from build123d import *

# Parameters (mm, degrees)
F3_DEPTH  = 5
F5_DEPTH  = 15
F6_W      = 2
F6_H      = 3
F7_DEPTH  = 20.5
F8_W      = 3
F8_H      = 1
F9_DEPTH  = 17.5068136575
F10_R     = 0.3
F11_R     = 0.1
F12_R     = 0.1
F13_W     = 100
F13_H     = 100
F14_DEPTH = 46.1004730675


with BuildPart() as f2:
    # F1 (on Front) → F2 (revolve)
    with BuildSketch(Plane.XZ):
        with BuildLine():
            Line((-2, 62), (-10, 62))
            add(Edge.make_bspline(
                [(-10, 62), (-11.8174263966, 57.1809415466), (-15.8594861297, 46.4373198499), (-18.6273544316, 24.5459471202), (-15.0414654734, -19.3469968059), (-5.4834802074, -38.7438846901), (-1.25, -47.0509425635)],
                knots=[0, 0, 0, 0, 0.1886807773, 0.4119593541, 0.7294893705, 0.9757699691, 0.9757699691, 0.9757699691, 0.9757699691], degree=3))
            Line((-1.25, -47.0509425635), (-1.25, -43.0509425635))
            Line((-1.25, -43.0509425635), (-1.75, -43.0509425635))
            Line((-1.75, -43.0509425635), (-1.75, -19.5))
            Line((-1.75, -19.5), (0, -19.5))
            Line((0, -19.5), (0, 47))
            Line((0, 47), (0, 50))
            Line((0, 50), (-2, 50))
            Line((-2, 50), (-2, 62))
        make_face()
    revolve(axis=Axis((0, 0, 54.5), (0, 0, 1)))

    # F0 (on Front) → F3 (cut, symmetric)
    with BuildSketch(Plane.XZ):
        Polygon((-10.75, -19.5), (10.75, -19.5), (10.75, 44.5), (9, 44.5), (9, 50.5), (-9, 50.5), (-9, 44.5), (-10.75, 44.5), align=None)
    extrude(amount=F3_DEPTH, both=True, mode=Mode.SUBTRACT)

    # F4 (on face) → F5 (cut)
    with BuildSketch(Plane.XY.offset(62)):
        Polygon((1.2421649551, -1.9468845774), (2.3071339798, 0.1023041181), (1.0649690247, 2.0491886955), (-1.2421649551, 1.9468845774), (-2.3071339798, -0.1023041181), (-1.0649690247, -2.0491886955), align=None)
    extrude(amount=-F5_DEPTH, mode=Mode.SUBTRACT)

    # F6 (on Right) → F7 (cut, symmetric)
    with BuildSketch(Plane.YZ):
        with Locations((-0.8976958819, 48.5)):
            Rectangle(F6_W, F6_H)
    extrude(amount=F7_DEPTH, both=True, mode=Mode.SUBTRACT)

    # F8 (on Front) → F9 (cut, through all)
    with BuildSketch(Plane.XZ):
        with Locations((0, 41.5)):
            Rectangle(F8_W, F8_H)
    extrude(amount=F9_DEPTH, mode=Mode.SUBTRACT)

    # F10
    f10_edges = [f2.edges().sort_by_distance(p)[0] for p in [
        (1.25, 0, -47.050943),
    ]]
    fillet(f10_edges, radius=F10_R)

    # F11
    f11_edges = [f2.edges().sort_by_distance(p)[0] for p in [
        (1.25, 0, -43.050943),
    ]]
    fillet(f11_edges, radius=F11_R)

    # F12
    f12_edges = [f2.edges().sort_by_distance(p)[0] for p in [
        (1.75, 0, -43.050943),
    ]]
    fillet(f12_edges, radius=F12_R)

    # F13 (on Top) → F14 (cut, through all)
    with BuildSketch(Plane.XY):
        Rectangle(F13_W, F13_H)
    extrude(amount=-F14_DEPTH, mode=Mode.SUBTRACT)


solid = f2.part
Geometry check sheet. Reference: the model listing, model coordinates, mm. A direction names the side the tool comes from. Round coordinates to 2 decimals unless told otherwise and drop trailing zeros.
Item 1: Material ranges on line 1 along Y through (x, z) = (0.5, 37.5); line 2 along Y through (x, z) = (-6.5, 4); line 3 along X through (y, z) = (4, 28), recorded low to high.
Determined:
line 1: y = -16.75 to -5, 5 to 16.75
line 2: y = -15.17 to -5, 5 to 15.17
line 3: x = -16.98 to -10.75, 10.75 to 16.98
Item 2: Access from +Z, -Z, +X, -X, +Y, -Y to the whole of each face (thin tool, end or side, straight path). Record for faces 1 (the face through (12, 0.102, 48)), 2 (the face through (-10.75, 0, 23)), 3 (the face through (0, -2, 56)).
Determined:
face 1: +X, -X
face 2: -Z
face 3: +Z, -Z
Item 3: Go/stop test with flat-tipped pins: pin 1 Ø10 at (y, z) = (5, 29) entering from -X; pin 2 Ø0.5 at (y, z) = (-12, 41.5) entering from -X; pin 3 Ø8 at (y, z) = (0.5, 30) entering from +X. Record where each tip stops, or that it passes through.
Determined:
pin 1: stops at x = -17.47
pin 2: stops at x = -11.12
pin 3: stops at x = 17.49
Item 4: Mould release check, pull along Y, two halves, no side actions. Record for faces 4 (the face through (0, -10, 42)), 5 (the face through (0, -5, 26)): +Y half, -Y half, draft (parallel to the pull), parting line (faces both ways), or undercut.
Determined:
face 4: draft
face 5: undercut
Item 5: Section check A-A (y = -1). Give the number of separate pieces and of enclosed holes in the cut face, plus the area to 3 significant figures.
Determined:
separate pieces: 4
enclosed holes: 0
area: 825 mm2
